Geometry: final body of the model. Coordinates: model frame, mm. Face numbers are marked on the shaded views. Give positions to 0.01 mm unless a question says otherwise; leave off trailing zeros. Order: outer loops, then holes, each group sorted by start corner. A loop starts at its lowest first (then second) coordinate and runs counter-clockwise, first axis right, second up. Notation, with made-up numbers: (81, -25.75) - (132, -25.75) arc R19 ccw to (132, 7.25) - close; hole circle Ø8 at (50.25, 44). An arc over 180 degrees is marked (long way). Write item = value, one per line. Start each with the question number.
from build123d import *

# Parameters (mm, degrees)
EXTRUDE001_DEPTH = 3
EXTRUDE_DEPTH    = 13
PAD_DEPTH        = 1


with BuildPart() as logo:
    # Clone001 → Extrude001 (new body)
    with BuildSketch(Plane(origin=(-0.02902, 0.352548, 0), x_dir=(0, 1, 0), z_dir=(0, 0, 1))):
        with BuildLine():
            Line((11.003952, 0), (11.003952, 4.6902))
            add(Edge.make_bspline(
                [(17.495532, 11.11494), (17.439852, 9.87498), (18.110958, 3.851298), (11.003952, 4.6902)],
                knots=[0, 0, 0, 0, 1, 1, 1, 1], degree=3))
            Line((17.495532, 11.11494), (17.495532, 13.69728))
            add(Edge.make_bspline(
                [(17.495532, 13.69728), (17.55828, 20.39472), (9.268146, 22.052754), (6.725322, 16.344462)],
                knots=[0, 0, 0, 0, 1, 1, 1, 1], degree=3))
            Line((6.725322, 16.344462), (3.636072, 10.55046))
            add(Edge.make_bspline(
                [(3.636072, 10.55046), (1.910148, 7.910058), (-1.368966, 7.43109), (-5.653788, 7.349202)],
                knots=[0, 0, 0, 0, 1, 1, 1, 1], degree=3))
            Line((-5.653788, 7.349202), (-10.55505, 7.349202))
            Line((-10.55505, 7.349202), (-10.55505, 19.368439))
            Line((-10.55505, 19.368439), (-4.848108, 19.368439))
            add(Edge.make_bspline(
                [(23.288592, 19.68918), (23.306112, 23.010726), (18.553098, 30.563958), (6.6153, 31.116642), (1.16223, 25.36881), (0.241104, 19.141998), (-4.848108, 19.368439)],
                knots=[0, 0, 0, 0, 0.25, 0.5, 0.75, 1, 1, 1, 1], degree=3))
            Line((23.288592, 19.68918), (23.288592, 8.37522))
            add(Edge.make_bspline(
                [(23.288592, 8.37522), (22.78257, 2.635146), (17.706012, 0)],
                knots=[0, 0, 0, 1, 1, 1], degree=2))
            add(Edge.make_bspline(
                [(23.288592, -8.37522), (22.78257, -2.635146), (17.706012, 0)],
                knots=[0, 0, 0, 1, 1, 1], degree=2))
            Line((23.288592, -8.37522), (23.288592, -19.68918))
            add(Edge.make_bspline(
                [(23.288592, -19.68918), (23.306112, -23.010726), (18.553098, -30.563958), (6.6153, -31.116642), (1.16223, -25.36881), (0.241104, -19.141998), (-4.848108, -19.23738)],
                knots=[0, 0, 0, 0, 0.25, 0.5, 0.75, 1, 1, 1, 1], degree=3))
            Line((-4.848108, -19.23738), (-10.55505, -19.23738))
            Line((-10.55505, -19.23738), (-10.55505, -7.463955))
            Line((-10.55505, -7.463955), (-5.653788, -7.463955))
            add(Edge.make_bspline(
                [(3.636072, -10.55046), (1.910148, -7.910058), (-1.368966, -7.43109), (-5.653788, -7.463955)],
                knots=[0, 0, 0, 0, 1, 1, 1, 1], degree=3))
            Line((3.636072, -10.55046), (6.725322, -16.344462))
            add(Edge.make_bspline(
                [(17.495532, -13.69728), (17.55828, -20.39472), (9.268146, -22.052754), (6.725322, -16.344462)],
                knots=[0, 0, 0, 0, 1, 1, 1, 1], degree=3))
            Line((17.495532, -13.69728), (17.495532, -11.11494))
            add(Edge.make_bspline(
                [(17.495532, -11.11494), (17.439852, -9.87498), (18.110958, -3.851298), (11.003952, -4.6902)],
                knots=[0, 0, 0, 0, 1, 1, 1, 1], degree=3))
            Line((11.003952, -4.6902), (11.003952, 0))
        make_face()
        with BuildLine():
            Line((-17.306112, 19.368439), (-16.106112, 19.368439))
            Line((-16.106112, 19.368439), (-16.106112, 7.349202))
            ThreePointArc((-16.106112, 7.349202), (-17.803168, 6.646258), (-18.506112, 4.949202))
            Line((-18.506112, 4.949202), (-18.506112, -5.063955))
            ThreePointArc((-18.506112, -5.063955), (-17.803168, -6.761011), (-16.106112, -7.463955))
            Line((-16.106112, -7.463955), (-16.106112, -19.23738))
            Line((-16.106112, -19.23738), (-23.306112, -19.23738))
            Line((-23.306112, -19.23738), (-23.306112, 13.368439))
            ThreePointArc((-23.306112, 13.368439), (-21.548753, 17.61108), (-17.306112, 19.368439))
        make_face()
    extrude(amount=EXTRUDE001_DEPTH)


with BuildPart() as basewall:
    # Sketch002 → Extrude (new body)
    with BuildSketch(Plane.XY):
        with BuildLine():
            Line((-46.351255, 34.299068), (-7.683758, 34.299068))
            Line((-7.683758, 36.699068), (-7.683758, 34.299068))
            Line((-47.208331, 36.699068), (-7.683758, 36.699068))
            ThreePointArc((-47.208331, 36.699068), (-48.905387, 35.996124), (-49.608331, 34.299068))
            Line((-49.608331, 29.202455), (-49.608331, 34.299068))
            Line((-49.608331, 29.202455), (-47.208331, 29.202455))
            Line((-47.208331, 29.202455), (-47.208331, 33.441992))
            ThreePointArc((-46.351255, 34.299068), (-46.957299, 34.048036), (-47.208331, 33.441992))
        make_face()
        with BuildLine():
            Line((46.991669, 33.796452), (46.991669, 29.202455))
            Line((46.991669, 29.202455), (49.391669, 29.202455))
            Line((49.391669, 34.299068), (49.391669, 29.202455))
            ThreePointArc((49.391669, 34.299068), (48.688725, 35.996124), (46.991669, 36.699068))
            Line((7.867758, 36.699068), (46.991669, 36.699068))
            Line((7.867758, 36.699068), (7.867758, 34.299068))
            Line((7.867758, 34.299068), (46.489053, 34.299068))
            ThreePointArc((46.991669, 33.796452), (46.844456, 34.151855), (46.489053, 34.299068))
        make_face()
        with BuildLine():
            Line((45.587676, -34.914826), (43.315151, -34.914826))
            Line((43.315151, -34.914826), (43.315152, -37.314826))
            Line((46.254463, -37.314826), (43.315152, -37.314826))
            ThreePointArc((46.254463, -37.314826), (48.472803, -36.395959), (49.391669, -34.177619))
            Line((49.391669, -12.051777), (49.391669, -34.177619))
            Line((46.991669, -12.051777), (49.391669, -12.051777))
            Line((46.991669, -12.051777), (46.991669, -33.510833))
            ThreePointArc((45.587676, -34.914826), (46.580449, -34.503606), (46.991669, -33.510833))
        make_face()
        with BuildLine():
            Line((-47.208331, -34.091189), (-47.208331, -12.051777))
            Line((-49.608331, -12.051777), (-47.208331, -12.051777))
            Line((-49.608331, -34.495377), (-49.608331, -12.051777))
            ThreePointArc((-49.608331, -34.495377), (-48.782534, -36.489028), (-46.788882, -37.314826))
            Line((-42.228662, -37.314826), (-46.788882, -37.314826))
            Line((-42.228662, -34.914826), (-42.228662, -37.314826))
            Line((-42.228662, -34.914826), (-46.384694, -34.914826))
            ThreePointArc((-47.208331, -34.091189), (-46.967093, -34.673588), (-46.384694, -34.914826))
        make_face()
        Polygon((-9.348882, -34.914826), (-9.348882, -37.314826), (5.543215, -37.314826), (5.543216, -34.914826), align=None)
    extrude(amount=EXTRUDE_DEPTH)


with BuildPart() as brandedbase:
    # Sketch → Pad (new body)
    with BuildSketch(Plane.XY):
        with BuildLine():
            Line((-47.208331, 36.699068), (46.991669, 36.699068))
            ThreePointArc((49.391669, 34.299068), (48.688725, 35.996124), (46.991669, 36.699068))
            Line((49.391669, 34.299068), (49.391669, -34.185399))
            ThreePointArc((46.257494, -37.314826), (48.472707, -36.399221), (49.391669, -34.185399))
            Line((46.257494, -37.314826), (-46.753742, -37.314826))
            ThreePointArc((-49.608331, -34.495164), (-48.765008, -36.4962), (-46.753742, -37.314826))
            Line((-49.608331, -34.495164), (-49.608331, 34.299068))
            ThreePointArc((-47.208331, 36.699068), (-48.905387, 35.996124), (-49.608331, 34.299068))
        make_face()
    extrude(amount=PAD_DEPTH)

    # Fusion: union BaseWall
    add(basewall.part)

    # Cut: cut Logo
    add(logo.part, mode=Mode.SUBTRACT)


solid = brandedbase.part
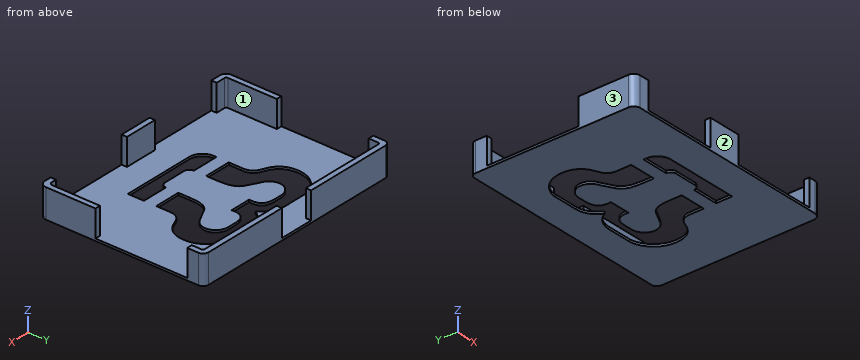
Q1. Pull-direction query (X, two-part tool) for the marked faces 1, 2 and 3; classes: +X half, -X half, draft (parallel to the pull), parting line (faces both ways), or undercut.
Q2. Section C-C, the plane x = -39.5. Return the cut outline in (y, z), then the cut area to 3 significant figures.
Q3. Material intervals for line 1 along X through (y, z) = (-21.5, 8.5); line 2 along Y through (x, z) = (43.5, 10); line 3 along Y through (x, z) = (-26, 1.25), sorted ascending. Write a range as from..to.
Q4. Section A-A, the plane y = -13.5. Return the cut outline in (x, z), then the cut area to 3 significant figures.
Q5. Contact query for flat-ended pins moving along their axis: pin 1 (2 mm diameter, centred on x = -34, y = -28, fed in from +Z); pin 2 (3 mm diameter, centred on x = -32.5, z = 10.5, fed in from -Y); pin 3 (2.5 mm diameter, centred on y = -36, z = 8.5, fed in from -X); pin 4 (1.9 mm diameter, centred on x = -48, z = 6, fed in from +Y). Output: stop coordinate, or through.
Q6. Section B-B, the plane z = 8.75. Count the separate pieces of the cut face and the enclosed holes in it, then the cut area to 3 significant figures.
The answers:
q1.face_1 = undercut
q1.face_2 = draft
q1.face_3 = -X half
q2.outline = (-37.31, 0) - (36.7, 0) - (36.7, 13) - (34.3, 13) - (34.3, 1) - (-37.31, 1) - close
q2.area = 103 mm²
q3.line_1 = -49.61..-47.21, 46.99..49.39
q3.line_2 = -37.31..-34.91, 34.3..36.7
q3.line_3 = 34.3..36.7
q4.outline = (-49.61, 0) - (49.39, 0) - (49.39, 13) - (46.99, 13) - (46.99, 1) - (-47.21, 1) - (-47.21, 13) - (-49.61, 13) - close
q4.area = 157 mm²
q5.pin_1 = 1
q5.pin_2 = 34.3
q5.pin_3 = -49.6
q5.pin_4 = 36.7
q6.separate_pieces = 5
q6.enclosed_holes = 0
q6.area = 397 mm²
